Read the model definition and answer for the solid it produces. Units are mm, in the model's axes. Coordinates: 2 decimals unless noted, no trailing zeros. Loops run counter-clockwise (first coordinate to the right, second up) from the corner with the lowest first, then second, coordinate; pieces in that order, holes last.
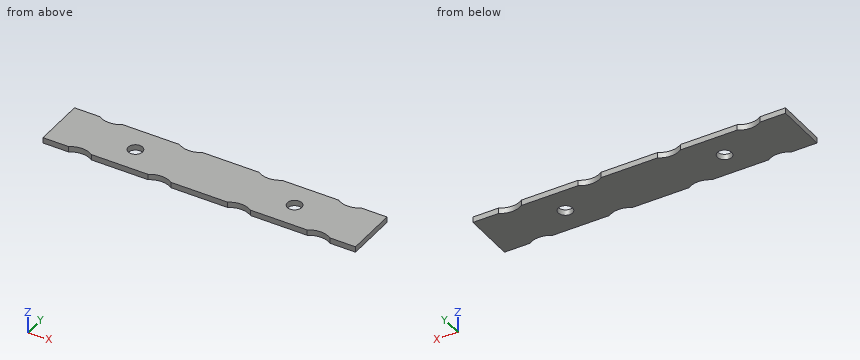
from build123d import *

# Parameters (mm, degrees)
SKETCH1_R           = 2.032
BOSS_EXTRUDE1_DEPTH = 1.6


with BuildPart() as part:
    # Sketch1 → Boss-Extrude1 (new body)
    with BuildSketch(Plane.XY):
        with BuildLine():
            Line((3.253099445, 19.430000002), (19.352900555, 19.430000002))
            ThreePointArc((19.352900555, 19.430000002), (22.606, 18.414000002), (25.859099445, 19.430000002))
            Line((25.859099445, 19.430000002), (41.958900555, 19.430000002))
            ThreePointArc((41.958900555, 19.430000002), (45.212, 18.414000002), (48.465099445, 19.430000002))
            Line((48.465099445, 19.430000002), (64.564900555, 19.430000002))
            ThreePointArc((64.564900555, 19.430000002), (67.818, 18.414000002), (71.071099445, 19.430000002))
            Line((71.071099445, 19.430000002), (78.318, 19.430000002))
            Line((78.318, 19.430000002), (78.318, 4.699999998))
            Line((78.318, 4.699999998), (71.071099445, 4.699999998))
            ThreePointArc((71.071099445, 4.699999998), (67.818, 5.715999998), (64.564900555, 4.699999998))
            Line((64.564900555, 4.699999998), (48.465099445, 4.699999998))
            ThreePointArc((48.465099445, 4.699999998), (45.212, 5.715999998), (41.958900555, 4.699999998))
            Line((41.958900555, 4.699999998), (25.859099445, 4.699999998))
            ThreePointArc((25.859099445, 4.699999998), (22.606, 5.715999998), (19.352900555, 4.699999998))
            Line((19.352900555, 4.699999998), (3.253099445, 4.699999998))
            ThreePointArc((3.253099445, 4.699999998), (0, 5.715999998), (-3.253099445, 4.699999998))
            Line((-3.253099445, 4.699999998), (-10.5, 4.699999998))
            Line((-10.5, 4.699999998), (-10.5, 19.430000002))
            Line((-10.5, 19.430000002), (-3.253099445, 19.430000002))
            ThreePointArc((-3.253099445, 19.430000002), (0, 18.414000002), (3.253099445, 19.430000002))
        make_face()
        with Locations((11.303, 12.065)):
            Circle(SKETCH1_R, mode=Mode.SUBTRACT)
        with Locations((56.515, 12.065)):
            Circle(SKETCH1_R, mode=Mode.SUBTRACT)
    extrude(amount=BOSS_EXTRUDE1_DEPTH)


solid = part.part
Item 1: A cutting plane is placed at A-A on z = 0.4. Determine the outline of the cut face in (x, y) (3 decimals).
Numbers:
outline: (-10.5, 4.7) - (-3.253, 4.7) arc R5.716 cw to (3.253, 4.7) - (19.353, 4.7) arc R5.716 cw to (25.859, 4.7) - (41.959, 4.7) arc R5.716 cw to (48.465, 4.7) - (64.565, 4.7) arc R5.716 cw to (71.071, 4.7) - (78.318, 4.7) - (78.318, 19.43) - (71.071, 19.43) arc R5.716 cw to (64.565, 19.43) - (48.465, 19.43) arc R5.716 cw to (41.959, 19.43) - (25.859, 19.43) arc R5.716 cw to (19.353, 19.43) - (3.253, 19.43) arc R5.716 cw to (-3.253, 19.43) - (-10.5, 19.43) - close; hole circle Ø4.064 at (11.303, 12.065); hole circle Ø4.064 at (56.515, 12.065)
Item 2: Find the intervals of material crossed by line 1 along X through (y, z) = (12.5, 0.65); line 2 along X through (y, z) = (13, 0.85); line 3 along Y through (x, z) = (11, 0.6), in increasing order.
Numbers:
line 1: x = -10.5 to 9.32, 13.29 to 54.53, 58.5 to 78.32
line 2: x = -10.5 to 9.5, 13.11 to 54.71, 58.32 to 78.32
line 3: y = 4.7 to 10.06, 14.07 to 19.43
Item 3: A cutting plane is placed at B-B on x = 65.5. Determine the outline of the cut face in (y, z).
Numbers:
outline: (5.22, 0) - (18.91, 0) - (18.91, 1.6) - (5.22, 1.6) - close
Item 4: Given pin 1 (2.5 mm diameter, centred on x = 11.303, y = 12.065, fed in from +Z), flat-ended and moving along its own axis, determine where the tip first touches the part or whether it passes through.
Numbers:
pin 1: passes through
Item 5: A cutting plane is placed at C-C on x = 45. Determine the outline of the cut face in (y, z), then the cut area to 3 significant figures.
Numbers:
outline: (5.71, 0) - (18.42, 0) - (18.42, 1.6) - (5.71, 1.6) - close
area: 20.3 mm2
